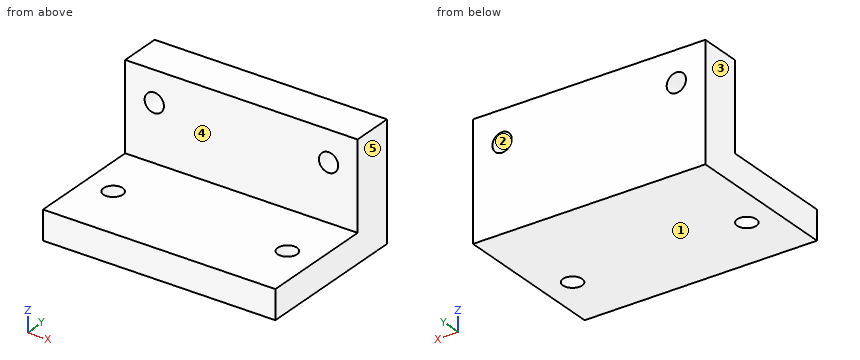
from build123d import *

# Parameters (mm, degrees)
SKETCH_1_W          = 80
SKETCH_1_H          = 40
EXTRUDE_1_DEPTH     = 10
SKETCH_4_R          = 3.32
CUT_EXTRUDE_3_DEPTH = 46.82575695
SKETCH_2_W          = 80
SKETCH_2_H          = 14.306395687
EXTRUDE_3_DEPTH     = 40
SKETCH_5_R          = 3.32
CUT_EXTRUDE_4_DEPTH = 40


with BuildPart() as part:
    # 草图1 → 凸台-拉伸1 (new body)
    with BuildSketch(Plane.XY):
        Rectangle(SKETCH_1_W, SKETCH_1_H)
    extrude(amount=EXTRUDE_1_DEPTH)

    # 草图4 → 切除-拉伸3 (cut, through all)
    with BuildSketch(Plane.XY.offset(10)):
        with Locations((30, 0)):
            Circle(SKETCH_4_R)
        with Locations((-30, 0)):
            Circle(SKETCH_4_R)
    extrude(amount=-CUT_EXTRUDE_3_DEPTH, mode=Mode.SUBTRACT)

    # 草图2 → 凸台-拉伸3 (add)
    with BuildSketch(Plane(origin=(0, 0, 0), x_dir=(-1, 0, 0), z_dir=(0, 0, -1))):
        with Locations((0, 27.153197844)):
            Rectangle(SKETCH_2_W, SKETCH_2_H)
    extrude(amount=-EXTRUDE_3_DEPTH)

    # 草图5 → 切除-拉伸4 (cut)
    with BuildSketch(Plane.XZ.offset(-20)):
        with Locations(Location((30, 29.40906451, 0), (0, 0, 270))):
            Circle(SKETCH_5_R)
        with Locations(Location((-30, 29.40906451, 0), (0, 0, 270))):
            Circle(SKETCH_5_R)
    extrude(amount=-CUT_EXTRUDE_4_DEPTH, mode=Mode.SUBTRACT)


solid = part.part
Geometry check sheet. Reference: the model listing, model coordinates, mm. Face numbers are marked on the shaded views. A direction names the side the tool comes from. Give positions to 0.01 mm unless a question says otherwise; leave off trailing zeros. Order: outer loops, then holes, each group sorted by start corner. A loop starts at its lowest first (then second) coordinate and runs counter-clockwise, first axis right, second up.
1. Draft check along Z on the marked faces 1, 2 and 3. Enter one of: pulls with the +Z half, pulls with the -Z half, needs draft (parallel to the pull), parting line crosses it, or undercut.
Completed:
face 1: pulls with the -Z half
face 2: undercut
face 3: needs draft
2. Sectioned sample at A-A (y = 0). Record the boundary of the cut face in (x, z), then the cut area to 3 significant figures.
Completed:
outline: (-40, 0) - (-33.32, 0) - (-33.32, 10) - (-40, 10) - close; (-26.68, 0) - (26.68, 0) - (26.68, 10) - (-26.68, 10) - close; (33.32, 0) - (40, 0) - (40, 10) - (33.32, 10) - close
area: 667 mm2
3. Depth check by flat-ended pin: pin 1 (8.5 mm diameter, centred on x = -30, z = 29.41, fed in from -Y); pin 2 (1 mm diameter, centred on x = -25, y = 17, fed in from +Z); pin 3 (6 mm diameter, centred on x = -30, y = 0, fed in from +Z). Enter the tip coordinate at first touch or a pass-through.
Completed:
pin 1: stops at y = 20
pin 2: stops at z = 10
pin 3: passes through
4. Access from +Z, -Z, +X, -X, +Y, -Y to the whole of each face (thin tool, end or side, straight path). Record for the marked faces 4 and 5.
Completed:
face 4: +Z, +X, -X, -Y
face 5: +Z, -Z, +X, +Y, -Y
5. Sectioned sample at D-D (z = 31.5). Record the boundary of the cut face in (x, y), then the cut area to 3 significant figures.
Completed:
outline: (-40, 20) - (-32.58, 20) - (-32.58, 34.31) - (-40, 34.31) - close; (-27.42, 20) - (27.42, 20) - (27.42, 34.31) - (-27.42, 34.31) - close; (32.58, 20) - (40, 20) - (40, 34.31) - (32.58, 34.31) - close
area: 997 mm2
6. Scan lines: line 1 (X direction, y = 22, z = 28); line 2 (Z direction, x = -16.5, y = 11); line 3 (Y direction, x = 30, z = 3). Record each from-to range of solid material in increasing order.
Completed:
line 1: x = -40 to -33.01, -26.99 to 26.99, 33.01 to 40
line 2: z = 0 to 10
line 3: y = -20 to -3.32, 3.32 to 34.31
7. Sectioned sample at B-B (x = 30). Record the boundary of the cut face in (y, z).
Completed:
outline: (-20, 0) - (-3.32, 0) - (-3.32, 10) - (-20, 10) - close; (3.32, 0) - (34.31, 0) - (34.31, 26.09) - (20, 26.09) - (20, 10) - (3.32, 10) - close; (20, 32.73) - (34.31, 32.73) - (34.31, 40) - (20, 40) - close
8. Sectioned sample at C-C (z = 5). Record the boundary of the cut face in (x, y).
Completed:
outline: (-40, -20) - (40, -20) - (40, 34.31) - (-40, 34.31) - close; hole circle Ø6.64 at (-30, 0); hole circle Ø6.64 at (30, 0)
